Source: CAD feature listing. Evaluate the final solid. Frame: model axes, mm. Face numbers are marked on the shaded views. A direction names the side the tool comes from. Coordinates: 2 decimals unless noted, no trailing zeros. Write each loop counter-clockwise with the first axis right and the second up, starting at its lowest first coordinate (ties: lowest second). Pieces come first, ordered by that corner, then holes. Notation, with made-up numbers: (-23, 35.25) -> (10, 35.25) arc R13 ccw to (10, 41.25) -> close; hole circle Ø8 at (8.5, 27.5). An arc over 180 degrees is marked (long way). One line per item, written item: value. Start each with the question number.
1. First-contact query: P1, Ø2, axis at x = -3.5, y = 4, coming from the -Z side; P2, Ø2.5, axis at x = 15.75, z = -21.96, coming from the +Y side; P3, Ø2, axis at x = -8, y = 2.5, coming from the -Z side. Flat tips, straight axial feed; report the tip coordinate or a pass-through.
2. Section query D-D, the plane z = -5. Output: boundary loops of the cut face in (x, y).
3. Section query A-A, the plane z = -22.5. Output: boundary loops of the cut face in (x, y).
4. Section query B-B, the plane y = 2.5. Output: boundary loops of the cut face in (x, z).
5. Mould query, pull axis X, two halves, no side actions, for the marked faces 1, 2, 3 and 4. Classes: released by +X, released by -X, zero draft, split by the parting line, or undercut.
6. Access query for the marked faces 5 and 6. Directions: +Z, -Z, +X, -X, +Y, -Y. A direction counts if a zero-diameter tool reaches every point of the face in a straight line with its end or side. Return the directions, or none.
7. Line query: line 1 (X direction, y = 3.05, z = -22); line 2 (Z direction, x = -13.5, y = 2.5); line 3 (Z direction, x = 22, y = 3.45). Output: solid intervals per line, ascending.
8. Section query C-C, the plane x = 0. Output: boundary loops of the cut face in (y, z), and give its area (3 significant figures).
from build123d import *

# Parameters (mm, degrees)
SKIZZE1_R                       = 2
AUFSATZ_LINEAR_AUSTRAGEN1_DEPTH = 5
VERRUNDUNG1_R                   = 19
VERRUNDUNG2_R                   = 20


with BuildPart() as part:
    # Skizze1 → Aufsatz-Linear austragen1 (new body)
    with BuildSketch(Plane(origin=(0, 0, 0), x_dir=(1, 0, 0), z_dir=(0, 1, 0))):
        with BuildLine():
            Line((32.174930969, -0.758710751), (25.406405474, 24.546237926))
            ThreePointArc((25.406405474, 24.546237926), (15.641921228, 31.961749958), (6.033920269, 24.344579298))
            Line((6.033920269, 24.344579298), (4.193711044, 16.842429276))
            Line((4.193711044, 16.842429276), (-18.224781404, 0.973862232))
            ThreePointArc((-18.224781404, 0.973862232), (-21.454022597, -11.53334461), (-9.654845468, -16.790495999))
            Line((-9.654845468, -16.790495999), (8.801061186, -11.423209418))
            Line((8.801061186, -11.423209418), (20.984655174, -13.357550953))
            ThreePointArc((20.984655174, -13.357550953), (30.029331036, -10.12200662), (32.174930969, -0.758710751))
        make_face()
        with Locations(Location((22.552676727, -3.481250613, 0), (0, 0, 270))):
            Circle(SKIZZE1_R, mode=Mode.SUBTRACT)
        with Locations(Location((-12.447323273, -7.188305222, 0), (0, 0, 270))):
            Circle(SKIZZE1_R, mode=Mode.SUBTRACT)
        with Locations(Location((15.746010972, 21.962291706, 0), (0, 0, 270))):
            Circle(SKIZZE1_R, mode=Mode.SUBTRACT)
    extrude(amount=AUFSATZ_LINEAR_AUSTRAGEN1_DEPTH)

    # Verrundung1
    verrundung1_edges = [part.edges().sort_by_distance(p)[0] for p in [
        (4.193711044, 2.5, -16.842429276),
    ]]
    fillet(verrundung1_edges, radius=VERRUNDUNG1_R)

    # Verrundung2
    verrundung2_edges = [part.edges().sort_by_distance(p)[0] for p in [
        (8.801061186, 2.5, 11.423209418),
    ]]
    fillet(verrundung2_edges, radius=VERRUNDUNG2_R)


solid = part.part
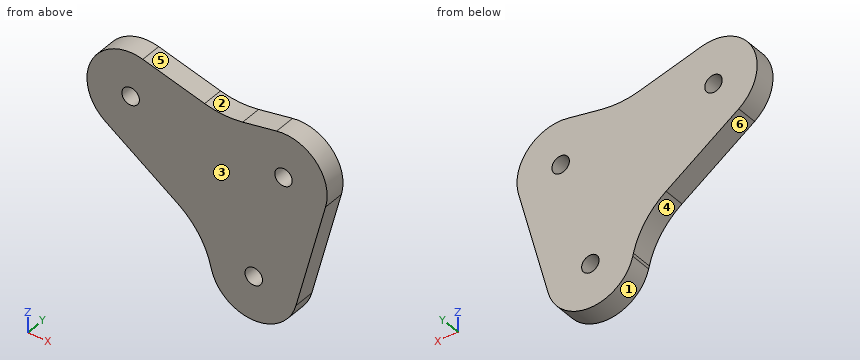
Computed values:
1. P1: stops at z = -12.1
1. P2: passes through
1. P3: stops at z = -8.92
2. outline: (-12.54, 0) -> (30.63, 0) -> (30.63, 5) -> (-12.54, 5) -> close
3. outline: (5.54, 0) -> (13.82, 0) -> (13.82, 5) -> (5.54, 5) -> close; (17.67, 0) -> (25.95, 0) -> (25.95, 5) -> (17.67, 5) -> close
4. outline: (-18.22, -0.97) -> (-1.59, -12.75) arc R19 cw to (5.88, -23.73) -> (6.03, -24.34) arc R10 ccw to (25.41, -24.55) -> (32.17, 0.76) arc R10 ccw to (20.98, 13.36) -> (13.22, 12.13) arc R20 cw to (4.5, 12.67) -> (-9.65, 16.79) arc R10 ccw to start; hole circle Ø4 at (-12.45, 7.19); hole circle Ø4 at (15.75, -21.96); hole circle Ø4 at (22.55, 3.48)
5. face 1: split by the parting line
5. face 2: undercut
5. face 3: zero draft
5. face 4: released by -X
6. face 5: +Z, +Y, -Y
6. face 6: -Z, -X, +Y, -Y
7. line 1: x = 5.37 to 13.75, 17.75 to 26.09
7. line 2: z = -4.32 to 5.49, 8.89 to 17.13
7. line 3: z = -29.77 to 1.56, 5.4 to 13.47
8. outline: (0, -14.01) -> (5, -14.01) -> (5, 13.98) -> (0, 13.98) -> close
8. area: 140 mm²
